Geometry: final body of the model. Coordinates: model frame, mm. Coordinates: 2 decimals unless noted, no trailing zeros. Write each loop counter-clockwise with the first axis right and the second up, starting at its lowest first coordinate (ties: lowest second). Pieces come first, ordered by that corner, then holes.
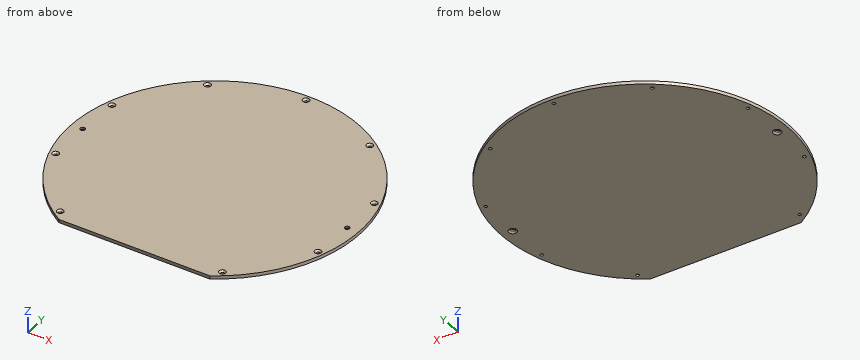
from build123d import *

# Parameters (mm, degrees)
RESSALTO_EXTRUS_O1_DEPTH = 2
CORTE_EXTRUS_O2_REACH    = 4
ESBO_O3_R                = 1.5
CHANFRO2_SIZE            = 1
CORTE_EXTRUS_O3_REACH    = 4
ESBO_O4_R                = 1
CHANFRO3_SIZE            = 1


with BuildPart() as part:
    # Esboço1 → Ressalto-extrusão1 (new body)
    with BuildSketch(Plane.XY):
        with BuildLine():
            Line((-46.303347611, -74.833147735), (46.303347611, -74.833147735))
            ThreePointArc((46.303347611, -74.833147735), (0, 88), (-46.303347611, -74.833147735))
        make_face()
    extrude(amount=RESSALTO_EXTRUS_O1_DEPTH)

    # Esboço3 → Corte-extrusão2 (cut, up to next)
    with BuildSketch(Plane.XY.offset(2), mode=Mode.PRIVATE) as corte_extrus_o2_sk1:
        with Locations((81, 0)):
            Circle(ESBO_O3_R)
    corte_extrus_o2_tool1 = extrude(corte_extrus_o2_sk1.sketch, amount=-CORTE_EXTRUS_O2_REACH, mode=Mode.PRIVATE) & part.part
    add(corte_extrus_o2_tool1.solids().sort_by_distance((81, 0, 2))[0], mode=Mode.SUBTRACT)
    # Esboço3 → Corte-extrusão2 (cut, up to next)
    with BuildSketch(Plane.XY.offset(2), mode=Mode.PRIVATE) as corte_extrus_o2_sk2:
        with Locations((-81, 0)):
            Circle(ESBO_O3_R)
    corte_extrus_o2_tool2 = extrude(corte_extrus_o2_sk2.sketch, amount=-CORTE_EXTRUS_O2_REACH, mode=Mode.PRIVATE) & part.part
    add(corte_extrus_o2_tool2.solids().sort_by_distance((-81, 0, 2))[0], mode=Mode.SUBTRACT)

    # Chanfro2
    chanfro2_edges = [part.edges().sort_by_distance(p)[0] for p in [
        (79.5, 0, 0),
        (-82.5, 0, 0),
    ]]
    chamfer(chanfro2_edges, length=CHANFRO2_SIZE)

    # Esboço4 → Corte-extrusão3 (cut, up to next)
    with BuildSketch(Plane.XY.offset(2), mode=Mode.PRIVATE) as corte_extrus_o3_sk1:
        with Locations((-49.667853819, -68.361936025)):
            Circle(ESBO_O4_R)
    corte_extrus_o3_tool1 = extrude(corte_extrus_o3_sk1.sketch, amount=-CORTE_EXTRUS_O3_REACH, mode=Mode.PRIVATE) & part.part
    add(corte_extrus_o3_tool1.solids().sort_by_distance((-49.667854, -68.361936, 2))[0], mode=Mode.SUBTRACT)
    # Esboço4 → Corte-extrusão3 (cut, up to next)
    with BuildSketch(Plane.XY.offset(2), mode=Mode.PRIVATE) as corte_extrus_o3_sk2:
        with Locations((-80.364275627, -26.111936025)):
            Circle(ESBO_O4_R)
    corte_extrus_o3_tool2 = extrude(corte_extrus_o3_sk2.sketch, amount=-CORTE_EXTRUS_O3_REACH, mode=Mode.PRIVATE) & part.part
    add(corte_extrus_o3_tool2.solids().sort_by_distance((-80.364276, -26.111936, 2))[0], mode=Mode.SUBTRACT)
    # Esboço4 → Corte-extrusão3 (cut, up to next)
    with BuildSketch(Plane.XY.offset(2), mode=Mode.PRIVATE) as corte_extrus_o3_sk3:
        with Locations((-80.364275627, 26.111936025)):
            Circle(ESBO_O4_R)
    corte_extrus_o3_tool3 = extrude(corte_extrus_o3_sk3.sketch, amount=-CORTE_EXTRUS_O3_REACH, mode=Mode.PRIVATE) & part.part
    add(corte_extrus_o3_tool3.solids().sort_by_distance((-80.364276, 26.111936, 2))[0], mode=Mode.SUBTRACT)
    # Esboço4 → Corte-extrusão3 (cut, up to next)
    with BuildSketch(Plane.XY.offset(2), mode=Mode.PRIVATE) as corte_extrus_o3_sk4:
        with Locations((-49.667853819, 68.361936025)):
            Circle(ESBO_O4_R)
    corte_extrus_o3_tool4 = extrude(corte_extrus_o3_sk4.sketch, amount=-CORTE_EXTRUS_O3_REACH, mode=Mode.PRIVATE) & part.part
    add(corte_extrus_o3_tool4.solids().sort_by_distance((-49.667854, 68.361936, 2))[0], mode=Mode.SUBTRACT)
    # Esboço4 → Corte-extrusão3 (cut, up to next)
    with BuildSketch(Plane.XY.offset(2), mode=Mode.PRIVATE) as corte_extrus_o3_sk5:
        with Locations((0, 84.5)):
            Circle(ESBO_O4_R)
    corte_extrus_o3_tool5 = extrude(corte_extrus_o3_sk5.sketch, amount=-CORTE_EXTRUS_O3_REACH, mode=Mode.PRIVATE) & part.part
    add(corte_extrus_o3_tool5.solids().sort_by_distance((0, 84.5, 2))[0], mode=Mode.SUBTRACT)
    # Esboço4 → Corte-extrusão3 (cut, up to next)
    with BuildSketch(Plane.XY.offset(2), mode=Mode.PRIVATE) as corte_extrus_o3_sk6:
        with Locations((49.667853819, 68.361936025)):
            Circle(ESBO_O4_R)
    corte_extrus_o3_tool6 = extrude(corte_extrus_o3_sk6.sketch, amount=-CORTE_EXTRUS_O3_REACH, mode=Mode.PRIVATE) & part.part
    add(corte_extrus_o3_tool6.solids().sort_by_distance((49.667854, 68.361936, 2))[0], mode=Mode.SUBTRACT)
    # Esboço4 → Corte-extrusão3 (cut, up to next)
    with BuildSketch(Plane.XY.offset(2), mode=Mode.PRIVATE) as corte_extrus_o3_sk7:
        with Locations((80.364275627, 26.111936025)):
            Circle(ESBO_O4_R)
    corte_extrus_o3_tool7 = extrude(corte_extrus_o3_sk7.sketch, amount=-CORTE_EXTRUS_O3_REACH, mode=Mode.PRIVATE) & part.part
    add(corte_extrus_o3_tool7.solids().sort_by_distance((80.364276, 26.111936, 2))[0], mode=Mode.SUBTRACT)
    # Esboço4 → Corte-extrusão3 (cut, up to next)
    with BuildSketch(Plane.XY.offset(2), mode=Mode.PRIVATE) as corte_extrus_o3_sk8:
        with Locations((80.364275627, -26.111936025)):
            Circle(ESBO_O4_R)
    corte_extrus_o3_tool8 = extrude(corte_extrus_o3_sk8.sketch, amount=-CORTE_EXTRUS_O3_REACH, mode=Mode.PRIVATE) & part.part
    add(corte_extrus_o3_tool8.solids().sort_by_distance((80.364276, -26.111936, 2))[0], mode=Mode.SUBTRACT)
    # Esboço4 → Corte-extrusão3 (cut, up to next)
    with BuildSketch(Plane.XY.offset(2), mode=Mode.PRIVATE) as corte_extrus_o3_sk9:
        with Locations((49.667853819, -68.361936025)):
            Circle(ESBO_O4_R)
    corte_extrus_o3_tool9 = extrude(corte_extrus_o3_sk9.sketch, amount=-CORTE_EXTRUS_O3_REACH, mode=Mode.PRIVATE) & part.part
    add(corte_extrus_o3_tool9.solids().sort_by_distance((49.667854, -68.361936, 2))[0], mode=Mode.SUBTRACT)

    # Chanfro3
    chanfro3_edges = [part.edges().sort_by_distance(p)[0] for p in [
        (-50.667853819, -68.361936025, 2),
        (-81.364275627, -26.111936025, 2),
        (-81.364275627, 26.111936025, 2),
        (-50.667853819, 68.361936025, 2),
        (-1, 84.5, 2),
        (48.667853819, 68.361936025, 2),
        (79.364275627, 26.111936025, 2),
        (79.364275627, -26.111936025, 2),
        (48.667853819, -68.361936025, 2),
    ]]
    chamfer(chanfro3_edges, length=CHANFRO3_SIZE)


solid = part.part
Item 1: Section C-C, the plane x = 36. Output: boundary loops of the cut face in (y, z), plus the area to 3 significant figures.
Derived:
outline: (-74.83, 0) - (80.3, 0) - (80.3, 2) - (-74.83, 2) - close
area: 310 mm2
Item 2: Material intervals for probe 1 along Y at (x, z) = (50.5, 1.9); probe 2 along Y at (x, z) = (-81, 1.3); probe 3 along X at (y, z) = (-25.5, 1.95), sorted ascending.
Derived:
probe 1: y = -72.07 to -70.07, -66.65 to 66.65, 70.07 to 72.07
probe 2: y = -34.39 to -27.25, -24.98 to -1.5, 1.5 to 24.98, 27.25 to 34.39
probe 3: x = -84.22 to -82.22, -78.51 to 78.51, 82.22 to 84.22
Item 3: Section B-B, the plane y = -56.5. Output: boundary loops of the cut face in (x, z).
Derived:
outline: (-67.47, 0) - (67.47, 0) - (67.47, 2) - (-67.47, 2) - close
Item 4: Pin query (flat end, axial travel): pin 1 (3 mm diameter, centred on x = -49.67, y = 68.36, fed in from +Z). Return the tip coordinate at first contact, or that it passes through.
Derived:
pin 1: stops at z = 1.5
Item 5: Section A-A, the plane z = 0.45. State how many separate pieces and enclosed holes the cut face has, plus the area to 3 significant figures.
Derived:
separate pieces: 1
enclosed holes: 11
area: 23,400 mm2
